Autodesk Inventor part; units mm, degrees
ref_plane "YZ Plane" through (0, 0, 0) normal (1, 0, 0) x (0, 1, 0)
ref_plane "XZ Plane" through (0, 0, 0) normal (0, 1, 0) x (-1, 0, 0)
ref_plane "XY Plane" through (0, 0, 0) normal (0, 0, 1) x (1, 0, 0)
sketch "Sketch1" plane through (0, 0, 0) normal (1, 0, 0) x (0, 1, 0)
  line L0 (0, 0) -> (160, 0)
  line L1 (160, 0) -> (160, -160)
  line L2 (160, -160) -> (0, -160)
  line L3 (0, -160) -> (0, 0)
  line L4 (0, 0) -> (5, 0)
  line L5 (5, 0) -> (5, -5)
  line L6 (5, -5) -> (0, -5)
  line L7 (0, -5) -> (0, 0)
  line L8 (5, -5) -> (155, -5)
  line L9 (155, -5) -> (155, -155)
  line L10 (155, -155) -> (5, -155)
  line L11 (5, -155) -> (5, -5)
  dimension "d0" = 160
  dimension "d1" = 160
  dimension "d2" = 5
  dimension "d3" = 5
  dimension "d4" = 150
  dimension "d5" = 150
extrude "Extrusion1" add sketch "Sketch1" along normal blind 10
sketch "Sketch2" plane through (10, 0, 0) normal (1, 0, 0) x (0, 0, -1)
  line L0 (5, 155) -> (155, 155)
  line L1 (5, 155) -> (10, 155)
  line L2 (10, 155) -> (10, 150)
  line L3 (10, 150) -> (5, 150)
  line L4 (5, 150) -> (5, 155)
  line L5 (10, 150) -> (150, 150)
  line L6 (150, 150) -> (150, 10)
  line L7 (150, 10) -> (10, 10)
  line L8 (10, 10) -> (10, 150)
  line L9 (160, 0) -> (160, 160)
  line L10 (0, 160) -> (160, 160)
  line L11 (160, 160) -> (160, 0)
  line L12 (160, 0) -> (0, 0)
  line L13 (0, 0) -> (0, 160)
  point P0 (0, 0)
  dimension "d8" = 5
  dimension "d9" = 5
  dimension "d10" = 140
  dimension "d11" = 140
extrude "Extrusion2" add sketch "Sketch2" along normal blind 4 contours L0 L2 L3 L4 | L12 L13 L10 L9
fillet "Fillet1" radius 10 4 edges at (5, 5, -155) (5, 155, -155) (5, 155, -5) (5, 5, -5)
fillet "Fillet2" radius 5 4 edges at (12, 10, -150) (12, 150, -150) (12, 10, -10) (12, 150, -10)
sketch "Sketch3" plane through (0, 0, 0) normal (-1, 0, 0) x (0, 0, 1)
  line L0 (-160, 160) -> (0, 160)
  line L1 (-160, 160) -> (0, 160) construction
  line L2 (-160, 150) -> (0, 150)
  line L3 (0, 170) -> (-160, 170)
  arc A0 (-160, 170) -> (-160, 150) centre (-160, 160) ccw
  arc A1 (0, 150) -> (0, 170) centre (0, 160) ccw
  line L4 (0, 160) -> (0, 0)
  line L5 (0, 0) -> (0, 160) construction
  line L6 (10, 0) -> (10, 160)
  line L7 (-10, 160) -> (-10, 0)
  arc A2 (-10, 0) -> (10, 0) centre (0, 0) ccw
  arc A3 (10, 160) -> (-10, 160) centre (0, 160) ccw
  line L8 (-160, 0) -> (-160, 160)
  line L9 (0, 0) -> (-160, 0) construction
  line L10 (0, 10) -> (-160, 10)
  line L11 (-160, -10) -> (0, -10)
  arc A4 (0, -10) -> (0, 10) centre (0, 0) ccw
  arc A5 (-160, 10) -> (-160, -10) centre (-160, 0) ccw
  line L12 (0, 0) -> (-160, 0)
  line L13 (-160, 0) -> (-160, 160) construction
  line L14 (-150, 0) -> (-150, 160)
  line L15 (-170, 160) -> (-170, 0)
  arc A6 (-170, 0) -> (-150, 0) centre (-160, 0) ccw
  arc A7 (-150, 160) -> (-170, 160) centre (-160, 160) ccw
  line L16 (-160, 160) -> (0, 160)
  line L17 (0, 160) -> (0, 0)
  line L18 (0, 0) -> (-160, 0)
  line L19 (-160, 0) -> (-160, 160)
  point P0 (-80, 160)
  point P1 (0, 80)
  point P2 (-80, 0)
  point P3 (-160, 80)
  point P4 (-170, 0)
  dimension "d16" = 10
extrude "Extrusion3" add sketch "Sketch3" against normal up to surface (14 mm away) contours L8 A0 A7 L0 | A7 L3 A3 L0 | L8 A5 L15 A0 | A3 A1 L4 L0 | L8 L12 A6 A5 | A1 L6 A4 L4 | L12 A2 L11 A6 | A4 A2 L12 L4
sketch "Sketch4" plane through (0, 0, 0) normal (-1, 0, 0) x (0, 0, 1)
  line L0 (-15, 150) -> (-145, 150)
  line L1 (-80, 150) -> (-80, 10)
  line L2 (-145, 10) -> (-15, 10)
  line L3 (-155.5, 4.5) -> (-4.5, 4.5)
  line L4 (-4.5, 4.5) -> (-4.5, 155.5)
  line L5 (-4.5, 155.5) -> (-155.5, 155.5)
  line L6 (-155.5, 155.5) -> (-155.5, 4.5)
  line L7 (-155.5, 4.5) -> (-4.5, 155.5) construction
  line L8 (-4.5, 4.5) -> (-155.5, 155.5) construction
  arc A0 (-145, 150) -> (-150, 145) centre (-145, 145) ccw
  circle A1 centre (-145, 145) radius 10.5
  arc A2 (-5, 145) -> (-15, 155) centre (-15, 145) ccw
  circle A3 centre (-15, 145) radius 10.5
  arc A4 (-15, 10) -> (-10, 15) centre (-15, 15) ccw
  circle A5 centre (-15, 15) radius 10.5
  arc A6 (-150, 15) -> (-145, 10) centre (-145, 15) ccw
  circle A7 centre (-145, 15) radius 10.5
  point P0 (0, 0)
  point P1 (-80, 80)
  point P2 (-4.5, 145)
  point P3 (-15, 155.5)
  point P4 (-145, 155.5)
  point P5 (-155.5, 145)
  point P6 (-155.5, 15)
  point P7 (-145, 4.5)
  point P8 (-15, 4.5)
  point P9 (-4.5, 15)
  dimension "d19" = 151
  dimension "d20" = 151
extrude "Extrusion4" cut sketch "Sketch4" against normal up to surface (10 mm away) contours A3 L4 A5 L2 L1 L0 | L0 A1 L5 A3 | A3 | L1 L2 A7 L6 A1 L0 | A1 | L2 A5 L3 A7 | A5 | A7
sketch "Sketch6" plane through (0, 0, 0) normal (-1, 0, 0) x (0, 0, 1)
  arc A0 (-145, 150) -> (-150, 145) centre (-145, 145) ccw
  circle A1 centre (-155.5, 155.5) radius 1.5
  circle A2 centre (-155.5, 155.5) radius 1.5
  arc A3 (-145, 155.5) -> (-155.5, 145) centre (-145, 145) ccw
  line L0 (-155.5, 155.5) -> (-145, 145)
  line L1 (-145, 145) -> (-155.5, 155.5)
  line L2 (-155.5, 155.5) -> (-158.5309, 158.5309)
  circle A4 centre (-145, 145) radius 17
  arc A5 (-10, 145) -> (-15, 150) centre (-15, 145) ccw
  line L3 (-145, 145) -> (-15, 145) construction
  line L4 (-145, 162) -> (-15, 162)
  line L5 (-15, 128) -> (-145, 128)
  arc A6 (-145, 162) -> (-145, 128) centre (-145, 145) ccw
  arc A7 (-15, 128) -> (-15, 162) centre (-15, 145) ccw
  arc A8 (-150, 15) -> (-145, 10) centre (-145, 15) ccw
  line L6 (-145, 145) -> (-145, 15) construction
  line L7 (-128, 145) -> (-128, 15)
  line L8 (-162, 15) -> (-162, 145)
  arc A9 (-128, 145) -> (-162, 145) centre (-145, 145) ccw
  arc A10 (-162, 15) -> (-128, 15) centre (-145, 15) ccw
  arc A11 (-15, 10) -> (-10, 15) centre (-15, 15) ccw
  line L9 (-145, 15) -> (-15, 15) construction
  line L10 (-145, 32) -> (-15, 32)
  line L11 (-15, -2) -> (-145, -2)
  arc A12 (-145, 32) -> (-145, -2) centre (-145, 15) ccw
  arc A13 (-15, -2) -> (-15, 32) centre (-15, 15) ccw
  line L12 (-15, 15) -> (-15, 145) construction
  line L13 (2, 15) -> (2, 145)
  line L14 (-32, 145) -> (-32, 15)
  arc A14 (-32, 15) -> (2, 15) centre (-15, 15) ccw
  arc A15 (2, 145) -> (-32, 145) centre (-15, 145) ccw
  line L15 (-180.2133, 180.2133) -> (20.1008, 180.2133)
  line L16 (20.1008, 180.2133) -> (20.1008, -29.1514)
  line L17 (20.1008, -29.1514) -> (-180.2133, -29.1514)
  line L18 (-180.2133, -29.1514) -> (-180.2133, 180.2133)
  point P0 (0, 0)
  point P1 (-80, 145)
  point P2 (-145, 80)
  point P3 (-80, 15)
  point P4 (-15, 80)
  point P5 (2, 145)
  point P6 (2, 15)
  point P7 (-145, -2)
  point P8 (-162, 145)
  point P9 (-145, 162)
  dimension "d26" = 10.5
  dimension "d27" = 10.5
  dimension "d28" = 34
  dimension "d38" = 164
  dimension "d39" = 17
  dimension "d43" = 17
  dimension "d44" = 17
extrude "Extrusion6" cut sketch "Sketch6" against normal blind 30 contours L15 L16 L17 L18
fillet "Fillet3" radius 6 4 edges at (14, 157.0208, -2.9792) (14, 2.9792, -2.9792) (14, 2.9792, -157.0208) (14, 157.0208, -157.0208)
chamfer "Chamfer1" distance 3 angle 45 4 edges at (14, 150, -80) (14, 80, -10) (14, 10, -80) (14, 80, -150)
fillet "Fillet4" radius 2 8 edges at (14, 150.6569, -150.6569) (14, 153, -80) (14, 150.6569, -9.3431) (14, 80, -7) (14, 9.3431, -9.3431) (14, 7, -80) (14, 9.3431, -150.6569) (14, 80, -153)
fillet "Fillet5" radius 1 8 edges at (11, 80, -150) (11, 11.4645, -148.5355) (11, 10, -80) (11, 11.4645, -11.4645) (11, 80, -10) (11, 148.5355, -11.4645) (11, 150, -80) (11, 148.5355, -148.5355)
fillet "Fillet6" radius 1 12 edges at (0, 152.4246, -152.4246) (0, 155.5, -80) (0, 152.4246, -7.5754) (0, 80, -4.5) (0, 7.5754, -7.5754) (0, 4.5, -80) (0, 7.5754, -152.4246) (0, 80, -155.5) (0, 2.9792, -157.0208) (0, 2.9792, -2.9792) (0, 157.0208, -2.9792) (0, 157.0208, -157.0208)
sketch "Sketch8" plane through (14, 0, 0) normal (1, 0, 0) x (0, 0, -1)
  line L0 (162, 15) -> (162, 145)
  line L1 (-2, 145) -> (-2, 15)
  line L2 (15, -2) -> (145, -2)
  line L3 (145, 162) -> (15, 162)
  line L4 (145, 155.5) -> (15, 155.5)
  point P0 (0, 0)
  dimension "d40" = 164
  dimension "d41" = 164
  dimension "d42" = 6.5
sketch "Sketch9" plane through (0, 0, 0) normal (-1, 0, 0) x (0, 0, 1)
  line L0 (-15, 150) -> (-145, 150)
  line L1 (-80, 150) -> (-80, 10)
  line L2 (-145, 10) -> (-15, 10)
  line L3 (-154.75, 5.25) -> (-5.25, 5.25)
  line L4 (-5.25, 5.25) -> (-5.25, 154.75)
  line L5 (-5.25, 154.75) -> (-154.75, 154.75)
  line L6 (-154.75, 154.75) -> (-154.75, 5.25)
  line L7 (-154.75, 5.25) -> (-5.25, 154.75) construction
  line L8 (-5.25, 5.25) -> (-154.75, 154.75) construction
  circle A0 centre (-154.75, 154.75) radius 1.6
  circle A1 centre (-5.25, 154.75) radius 1.6
  circle A2 centre (-154.75, 5.25) radius 1.6
  circle A3 centre (-5.25, 5.25) radius 1.6
  point P0 (0, 0)
  point P1 (-145, 145)
  point P2 (-15, 15)
  point P3 (-80, 80)
  dimension "d48" = 149.5
  dimension "d49" = 149.5
  dimension "d50" = 3.2
extrude "Extrusion7" cut sketch "Sketch9" against normal blind 10 contours L6 A2 L3 | L3 A2 L6 | A3 L4 L3 | L3 L4 A3 | A0 L5 L6 | L6 L5 A0 | A1 L5 L4 | L4 L5 A1
sketch "Sketch10" plane through (8, 15, 2) normal (0, 0, 1) x (1, 0, 0)
  line L0 (6, 0) -> (6, 130)
  line L1 (-8, 130) -> (-8, 0)
  line L2 (0, 130) -> (0, 0)
  point P0 (-8, -15)
  dimension "d53" = 14
  dimension "d54" = 8
sketch "Sketch11" plane through (10, 0, 0) normal (-1, 0, 0) x (0, 0, 1)
  line L0 (-145, 10) -> (-15, 10)
  line L1 (-15, 150) -> (-145, 150)
  line L2 (-15, 4.5) -> (-145, 4.5)
  line L3 (-145, 155.5) -> (-15, 155.5)
  line L4 (-80, 150) -> (-80, 10)
  line L5 (-7, 7) -> (-153, 7)
  line L6 (-153, 7) -> (-153, 153)
  line L7 (-153, 153) -> (-7, 153)
  line L8 (-7, 153) -> (-7, 7)
  line L9 (-7, 7) -> (-153, 153) construction
  line L10 (-153, 7) -> (-7, 153) construction
  point P0 (0, 0)
  point P1 (-80, 80)
  dimension "d55" = 140
  dimension "d56" = 151
  dimension "d57" = 146
  dimension "d58" = 146
chamfer "Chamfer2" distance 0.3 angle 45 4 edges at (0, 154.75, -6.85) (0, 154.75, -156.35) (0, 5.25, -156.35) (0, 5.25, -6.85)
sketch "Sketch17" plane through (14, 0, 0) normal (1, 0, 0) x (0, 0, -1)
  line L0 (-21.1254, 169.9507) -> (180.25, 169.9507)
  line L1 (180.25, 169.9507) -> (180.25, -9.9186)
  line L2 (180.25, -9.9186) -> (-21.1254, -9.9186)
  line L3 (-21.1254, -9.9186) -> (-21.1254, 169.9507)
  point P0 (0, 0)
extrude "Extrusion8" cut sketch "Sketch17" against normal blind 1.5
fillet "Fillet7" radius 3 16 edges at (12.5, 159.9686, -80) (12.5, 155.5844, -155.5844) (12.5, 80, -159.9686) (12.5, 4.4156, -155.5844) (12.5, 0.0314, -80) (12.5, 4.4156, -4.4156) (12.5, 80, -0.0314) (12.5, 155.5844, -4.4156) (12.5, 80, -8.5) (12.5, 10.4038, -10.4038) (12.5, 8.5, -80) (12.5, 10.4038, -149.5962) (12.5, 80, -151.5) (12.5, 149.5962, -149.5962) (12.5, 151.5, -80) (12.5, 149.5962, -10.4038)
sketch "Sketch18" plane through (0, 0, 0) normal (-1, 0, 0) x (0, 0, 1)
  line L0 (-183.9063, 166.801) -> (38.1322, 166.801)
  line L1 (38.1322, 166.801) -> (38.1322, -27.1199)
  line L2 (38.1322, -27.1199) -> (-183.9063, -27.1199)
  line L3 (-183.9063, -27.1199) -> (-183.9063, 166.801)
  point P0 (0, 0)
extrude "Extrusion9" cut sketch "Sketch18" against normal blind 1
fillet "Fillet8" radius 1 16 edges at (1, 80, -155.5) (1, 152.4246, -152.4246) (1, 155.5, -80) (1, 152.4246, -7.5754) (1, 80, -4.5) (1, 7.5754, -7.5754) (1, 4.5, -80) (1, 7.5754, -152.4246) (1, 2.9792, -157.0208) (1, -2, -80) (1, 2.9792, -2.9792) (1, 80, 2) (1, 157.0208, -2.9792) (1, 162, -80) (1, 157.0208, -157.0208) (1, 80, -162)
chamfer "Chamfer3" distance 0.3 angle 45 4 edges at (1, 5.25, -156.35) (1, 154.75, -156.35) (1, 154.75, -6.85) (1, 5.25, -6.85)
properties part number "DiffuserRetainer"
Part model, mm, in its own coordinate system. A direction names the side the tool comes from. Give positions to 0.01 mm unless a question says otherwise; leave off trailing zeros. Write each loop counter-clockwise with the first axis right and the second up, starting at its lowest first coordinate (ties: lowest second). Pieces come first, ordered by that corner, then holes.
1) Cut at A-A on z = -20.5. Write the cut outline in (x, y).
Resolved:
outline: (1, -1) arc R1 ccw to (2, -2) - (8, -2) arc R6 ccw to (11, -1.2) arc R3 ccw to (12.5, 1.4) - (12.5, 7.26) arc R3 ccw to (11.62, 9.38) - (11.29, 9.71) arc R1 ccw to (10.59, 10) - (10, 10) - (10, 4.5) - (2, 4.5) arc R1 ccw to (1, 3.5) - close; (1, 156.5) arc R1 ccw to (2, 155.5) - (10, 155.5) - (10, 150) - (10.59, 150) arc R1 ccw to (11.29, 150.29) - (11.62, 150.62) arc R3 ccw to (12.5, 152.74) - (12.5, 158.6) arc R3 ccw to (11, 161.2) arc R6 ccw to (8, 162) - (2, 162) arc R1 ccw to (1, 161) - close
2) Cut at C-C on x = 6. Write the cut outline in (y, z).
Resolved:
outline: (-2, -145) arc R17 ccw to (15, -162) - (145, -162) arc R17 ccw to (162, -145) - (162, -15) arc R17 ccw to (145, 2) - (15, 2) arc R17 ccw to (-2, -15) - close; hole circle Ø3.2 at (5.25, -154.75); hole circle Ø3.2 at (5.25, -5.25); hole (4.5, -145) arc R10.5 ccw to (15, -155.5) - (145, -155.5) arc R10.5 ccw to (155.5, -145) - (155.5, -15) arc R10.5 ccw to (145, -4.5) - (15, -4.5) arc R10.5 ccw to (4.5, -15) - close; hole circle Ø3.2 at (154.75, -154.75); hole circle Ø3.2 at (154.75, -5.25)
3) Probe L1, parallel to Y at x = 2.75, z = -120; L2, parallel to Z at x = 5.75, y = 43; L3, parallel to X at y = 154.5, z = -97.5. List the from-to ranges inside material, lowest first.
Resolved:
L1: y = -2 to 4.5, 155.5 to 162
L2: z = -162 to -155.5, -4.5 to 2
L3: x = 10 to 12.5
4) Two-plate mould, pull along Z, no slides. Class faces 1 (the face through (10, 8, -80)), 2 (the face through (4.96, 2.85, -3.11)), 3 (the face through (5, -2, -79)): released by +Z, released by -Z, zero draft, split by the parting line, or undercut.
Resolved:
face 1: undercut
face 2: released by +Z
face 3: zero draft
5) Pin check, flat tips, straight feed: pin 1 (0.6 mm diameter, centred on x = 10.5, y = 97, fed in from -Z); pin 2 (0.5 mm diameter, centred on x = 10.5, y = 110, fed in from +Z); pin 3 (1 mm diameter, centred on y = 4.5, z = -5, fed in from -X). Stop position of each tip, or through.
Resolved:
pin 1: stops at z = -161.58
pin 2: stops at z = 1.56
pin 3: stops at x = 10
6) Cut at B-B on y = 34.5. Write the cut outline in (x, z), then the cut area to 3 significant figures.
Resolved:
outline: (1, -161) arc R1 ccw to (2, -162) - (8, -162) arc R6 ccw to (11, -161.2) arc R3 ccw to (12.5, -158.6) - (12.5, -152.74) arc R3 ccw to (11.62, -150.62) - (11.29, -150.29) arc R1 ccw to (10.59, -150) - (10, -150) - (10, -155.5) - (2, -155.5) arc R1 ccw to (1, -156.5) - close; (1, -3.5) arc R1 ccw to (2, -4.5) - (10, -4.5) - (10, -10) - (10.59, -10) arc R1 ccw to (11.29, -9.71) - (11.62, -9.38) arc R3 ccw to (12.5, -7.26) - (12.5, -1.4) arc R3 ccw to (11, 1.2) arc R6 ccw to (8, 2) - (2, 2) arc R1 ccw to (1, 1) - close
area: 167 mm2
7) Which spindle directions (+Z, -Z, +X, -X, +Y, -Y) get a long thin tool onto all of the face, cutting with end or side? Do faces 4 (the face through (10.3, 11.43, -148.5)), 5 (the face through (11.423, 11.123, -148.792)), 6 (the face through (6, 79, -4.5)). Say none if no direction does.
Resolved:
face 4: +X, -X
face 5: +X
face 6: -X
